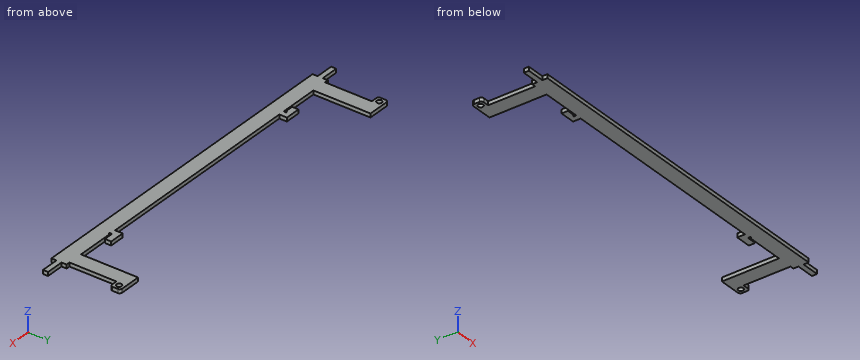
Autodesk Inventor part; units mm, degrees
ref_plane "YZ Plane" through (0, 0, 0) normal (1, 0, 0) x (0, 1, 0)
ref_plane "XY Plane" through (0, 0, 0) normal (0, 0, 1) x (1, 0, 0)
ref_plane "工作平面1" through (0, 0, 1.5) normal (0, 0, 1) x (1, 0, 0)
sketch "草圖1" plane through (0, 0, 0) normal (0, 0, 1) x (1, 0, 0)
  line L0 (0, 6) -> (0, -6)
  line L1 (0, -6) -> (-136, -6)
  line L2 (-136, -6) -> (-136, 6)
  line L3 (-150, 2) -> (-136, 2)
  line L4 (-136, 2) -> (-136, -2)
  line L5 (-136, -2) -> (-150, -2)
  line L6 (-150, -2) -> (-150, 2)
  line L7 (-210, 0) -> (210, 0)
  line L8 (0, -17.4828) -> (0, 62.8971)
  line L9 (0, -6) -> (136, -6)
  line L10 (136, -6) -> (136, 6)
  line L11 (150, 2) -> (136, 2)
  line L12 (136, -2) -> (150, -2)
  line L13 (150, -2) -> (150, 2)
  line L14 (136, -6) -> (136, -2)
  line L15 (145, 2) -> (139, 2)
  line L16 (-97.5, 7) -> (-97.5, 12)
  line L17 (-91, 7) -> (-97.5, 7)
  line L18 (97.5, 7) -> (97.5, 12)
  line L19 (97.5, 12) -> (87.5, 12)
  line L20 (90, 7) -> (97.5, 7)
  line L21 (90, 7) -> (90, 5)
  line L22 (90, 5) -> (91, 5)
  line L23 (91, 5) -> (91, 6)
  line L24 (-136, 6) -> (-91, 6)
  line L25 (-85.5, 6) -> (85.5, 6)
  line L26 (91, 6) -> (136, 6)
  line L27 (-85.5, 12) -> (-85.5, 6)
  line L28 (87.5, 12) -> (85.5, 12)
  line L29 (85.5, 12) -> (85.5, 6)
  line L30 (-97.5, 12) -> (-85.5, 12)
  line L31 (-91, 7) -> (-91, 8)
  line L32 (-91, 8) -> (-90, 8)
  line L33 (-90, 8) -> (-90, 7)
  line L34 (-90, 7) -> (-90, 6)
  line L35 (-91, 6) -> (-90, 6)
  point P0 (0, 0)
  point P1 (-136, 2)
  point P2 (136, -6)
  point P3 (136, -2)
  dimension "d2" = 4
  dimension "d14" = 2
  dimension "d17" = 12
  dimension "d57" = 14
  dimension "d58" = 300
  dimension "d62" = 2
  dimension "d63" = 85.5
  dimension "d64" = 85.5
  dimension "d65" = 12
  dimension "d66" = 5
  dimension "d67" = 6
  dimension "d68" = 6.5
  dimension "d69" = 136
  dimension "d70" = 14
  dimension "d71" = 136
  dimension "d72" = 272
extrude "擠出1" add sketch "草圖1" along normal blind 3
ref_plane "工作平面1" through (0, 0, 1.5) normal (0, 0, 1) x (1, 0, 0)
sketch "草圖7" plane through (0, 0, 0) normal (0, 0, -1) x (-1, 0, 0)
  line L0 (-210, 0) -> (210, 0)
  circle A0 centre (129.5, 0) radius 12.5
  line L1 (150, -2) -> (136, -2)
  line L2 (142, -2) -> (142, 2)
  line L3 (136, 2) -> (150, 2)
  line L4 (150, 2) -> (150, -2)
  circle A1 centre (129.5, 0) radius 2.05
  line L5 (136, 6) -> (136, 2)
  point P0 (0, 0)
  dimension "d36" = 25
  dimension "d38" = 4.1
  dimension "d73" = 6
extrude "擠出5" cut sketch "草圖7" against normal up to surface (3 mm away) contours A1 L0 | L0 A1
sketch "草圖8" plane through (0, 0, 3) normal (0, 0, 1) x (1, 0, 0)
  line L0 (-90, 6) -> (-136, 6)
  line L1 (-133, 6) -> (-121, 6)
  line L2 (-121, 6) -> (-121, 51)
  line L3 (-121, 51) -> (-136, 51)
  line L4 (-133, 43) -> (-133, 6)
  line L5 (-136, 6) -> (-136, 2)
  line L6 (-136, 51) -> (-139.5, 51)
  line L7 (-139.5, 51) -> (-139.5, 43)
  line L8 (-139.5, 43) -> (-133, 43)
  circle A0 centre (-135.5, 47) radius 2.05
  circle A1 centre (-129.5, 0) radius 2.05
  circle A2 centre (-135.5, 47) radius 6.5 construction
  line L9 (-136, 2) -> (-150, 2)
  line L10 (-150, 2) -> (-150, 58.0765) construction
  line L11 (-150, 58.0765) -> (-142, 58.0765) construction
  line L12 (-142, 58.0765) -> (-142, 42.2693) construction
  line L13 (-137.3204, 6) -> (-133, 6)
  line L14 (-133, 6) -> (-133, 16.271)
  circle A3 centre (-129.5, 16.6771) radius 2.05
  circle A4 centre (-129.5, 16.6771) radius 12.5 construction
  point P0 (0, 0)
  point P1 (-91, 6)
  dimension "d55" = 25
  dimension "d41" = 3
  dimension "d42" = 15
  dimension "d43" = 45
  dimension "d45" = 8
  dimension "d50" = 13
  dimension "d51" = 47
  dimension "d52" = 6.5
  dimension "d74" = 6
extrude "擠出6" add sketch "草圖8" against normal up to surface (3 mm away) contours L0 L4 L8 L7 L6 L3 L2 | A1 | A3
fillet "圓角2" radius 2 2 edges at (-139.5, 51, 1.5) (-139.5, 43, 1.5)
mirror "鏡射6" about plane through (0, 0, 0) normal (1, 0, 0) of "擠出5", "擠出6", "圓角2"
properties part number "rod_2" material "密集板"
Could you check a few things on this model? Use its own coordinates, in mm. Round coordinates to 2 decimals unless told otherwise and drop trailing zeros. Loops run counter-clockwise (first coordinate to the right, second up) from the corner with the lowest first, then second, coordinate; pieces in that order, holes last. Notation, with made-up numbers: M 58.5,-4 L 83.5,-4 A19 ccw 83.5,19 Z; hole C -34,54.5 d4. An arc over 180 degrees is marked long. Put each result on its own line as item: value.
Q1. Imagine slicing it at B-B (x = -33). Write out the boundary of the cut face in (y, z), then the cut area to 3 significant figures.
Check result:
outline: M -6,0 L 6,0 L 6,3 L -6,3 Z
area: 36.0 mm2
Q2. I need wall thicknesses on probe 1 along Y at (x, z) = (-135.5, 2.35); probe 2 along X at (y, z) = (9, 0.45); probe 3 along Y at (x, z) = (-94, 2.5). Which ranges of each line are inside material? Lowest first, please.
Check result:
probe 1: -6 to 6, 43 to 44.95, 49.05 to 51
probe 2: -133 to -121, -97.5 to -85.5, 85.5 to 97.5, 121 to 133
probe 3: -6 to 6, 7 to 12
Q3. Imagine slicing it at A-A (y = 30.5). Write out the boundary of the cut face in (x, z).
Check result:
outline: M -133,0 L -121,0 L -121,3 L -133,3 Z; M 121,0 L 133,0 L 133,3 L 121,3 Z
Q4. For pin 1 (1.1 mm diameter, centred on x = 90.5, z = 2, fed in from +Y); pin 2 (6 mm diameter, centred on x = -78, y = 11.5, fed in from +Z); pin 3 (0.9 mm diameter, centred on y = 4.5, z = 2, fed in from +X); pin 4 (1 mm diameter, centred on y = 19.5, z = 1, fed in from +X), each with a flat end and sliding along its axis, tell me the tip position at first contact or that it passes through.
Check result:
pin 1: y = 12
pin 2: through
pin 3: x = 136
pin 4: x = 133
Q5. Imagine slicing it at C-C (z = 2.15). State how many separate pieces and enclosed holes the cut face has, then the cut area to 3 significant figures.
Check result:
separate pieces: 1
enclosed holes: 2
area: 4,660 mm2
